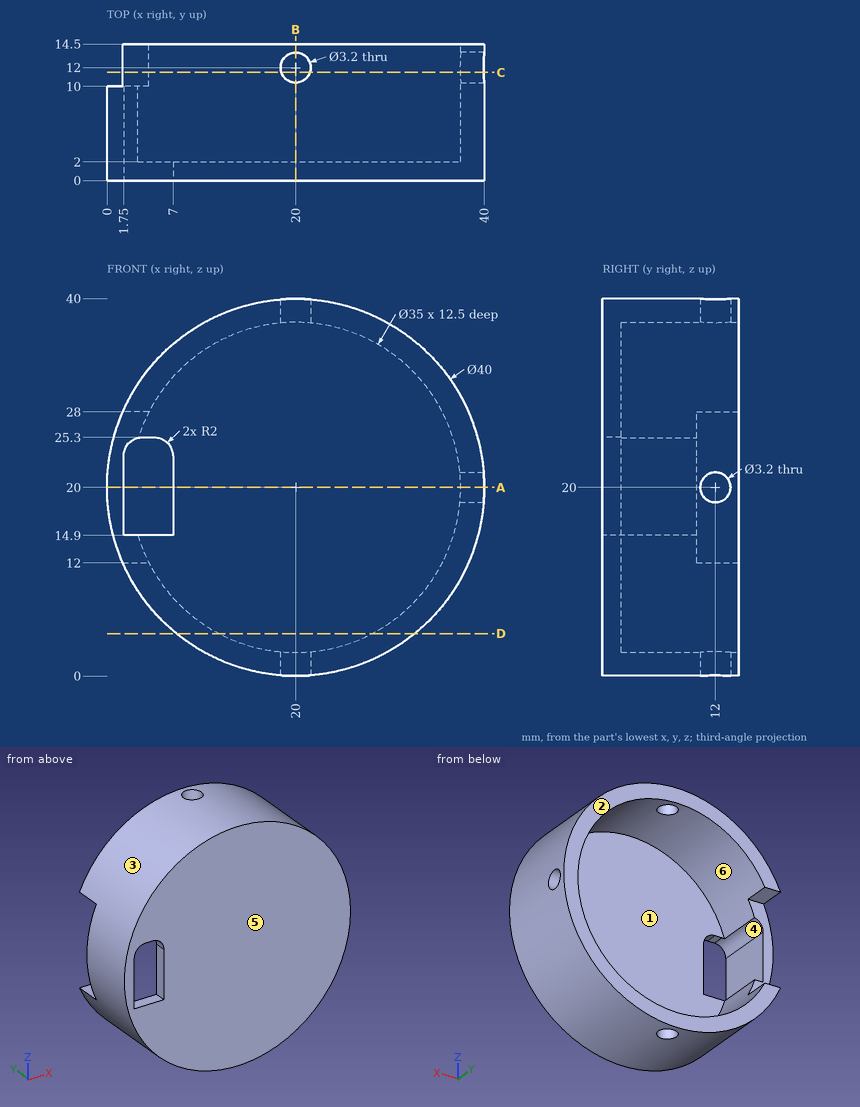
Verification items for this drawing (mm, ordinates from the low corner). A direction names the side the tool comes from. Coordinates: 2 decimals unless noted, no trailing zeros. Order: outer loops, then holes, each group sorted by start corner. A loop starts at its lowest first (then second) coordinate and runs counter-clockwise, first axis right, second up. Notation, with made-up numbers: M -12,74.5 L 19,74.5 A31 ccw 19,107.5 Z; hole C -16,-39.5 d5. An arc over 180 degrees is marked long. Answer as a JSON object with one key per item and string values.
Q1. Cross-section at D-D on z = 4.5. Record the cut outline in (x, y).
Results are:
{"outline": "M 7.36,0 L 32.64,0 L 32.64,14.5 L 28.12,14.5 L 28.12,2 L 11.88,2 L 11.88,14.5 L 7.36,14.5 Z"}
Q2. Cross-section at A-A on z = 20. Record the cut outline in (x, y).
Results are:
{"outline": "M 0,0 L 1.75,0 L 1.75,10 L 0,10 Z; M 7,0 L 40,0 L 40,10.4 L 37.5,10.4 L 37.5,2 L 7,2 Z; M 37.5,13.6 L 40,13.6 L 40,14.5 L 37.5,14.5 Z"}
Q3. Cross-section at C-C on y = 11.5. Record the cut outline in (x, z).
Results are:
{"outline": "M 1.67,12 A20 ccw 18.48,0.06 L 18.48,2.57 A17.5 cw 4.44,12 Z; M 1.67,28 L 4.44,28 A17.5 cw 18.48,37.43 L 18.48,39.94 A20 ccw Z; M 21.52,0.06 A20 ccw 39.94,18.48 L 37.43,18.48 A17.5 cw 21.52,2.57 Z; M 21.52,37.43 A17.5 cw 37.43,21.52 L 39.94,21.52 A20 ccw 21.52,39.94 Z"}
Q4. Scan lines: line 1 (Y direction, x = 20, z = 1.15); line 2 (Y direction, x = 17, z = 17); line 3 (Z direction, x = 3, y = 2). Record each from-to range of solid material in increasing order.
Results are:
{"line 1": "y = 0 to 10.4, 13.6 to 14.5", "line 2": "y = 0 to 2", "line 3": "z = 9.46 to 14.9, 25.15 to 30.54"}
Q5. Tool access check on the marked faces 4, 5 and 6. Record the directions out of +Z, -Z, +X, -X, +Y, -Y that give a thin tool (end or side, any length) a straight path to the whole face; none if there is none.
Results are:
{"face 4": "+Y, -Y", "face 5": "+Z, -Z, +X, -X, -Y", "face 6": "+Y"}
Q6. Depth check by flat-ended pin: pin 1 Ø1.4 at (x, y) = (2.5, 12.5) entering from +Z; pin 2 Ø1.4 at (x, y) = (2.5, 12) entering from -Z; pin 3 Ø8 at (y, z) = (9, 9.5) entering from +X; pin 4 Ø1.9 at (x, y) = (20, 12) entering from +Z. Enter the tip coordinate at first touch or a pass-through.
Results are:
{"pin 1": "stops at z = 30.85", "pin 2": "stops at z = 9.15", "pin 3": "stops at x = 38.91", "pin 4": "passes through"}
Q7. Cross-section at B-B on x = 20. Record the cut outline in (y, z).
Results are:
{"outline": "M 0,0 L 10.4,0 L 10.4,2.5 L 2,2.5 L 2,37.5 L 10.4,37.5 L 10.4,40 L 0,40 Z; M 13.6,0 L 14.5,0 L 14.5,2.5 L 13.6,2.5 Z; M 13.6,37.5 L 14.5,37.5 L 14.5,40 L 13.6,40 Z"}
Q8. Release check for a two-part mould opening along Z. For the marked faces 1, 2 and 3 record: released by +Z, released by -Z, zero draft, split by the parting line, or undercut.
Results are:
{"face 1": "undercut", "face 2": "zero draft", "face 3": "split by the parting line"}
